Geometry check sheet. Reference: the model listing, model coordinates, mm. A direction names the side the tool comes from. Give positions to 0.01 mm unless a question says otherwise; leave off trailing zeros. Order: outer loops, then holes, each group sorted by start corner. A loop starts at its lowest first (then second) coordinate and runs counter-clockwise, first axis right, second up.
Autodesk Inventor part; units mm, degrees
ref_plane "YZ Plane" through (0, 0, 0) normal (1, 0, 0) x (0, 1, 0)
ref_plane "XZ Plane" through (0, 0, 0) normal (0, 1, 0) x (-1, 0, 0)
ref_plane "XY Plane" through (0, 0, 0) normal (0, 0, 1) x (1, 0, 0)
sketch "スケッチ1" plane through (0, 0, 0) normal (0, 0, 1) x (1, 0, 0)
  circle A0 centre (0, 0) radius 35
  circle A1 centre (0, 0) radius 33
  line L0 (-45, 40) -> (45, 40)
  line L1 (45, 40) -> (45, -40)
  line L2 (45, -40) -> (-45, -40)
  line L3 (-45, -40) -> (-45, 40)
  line L4 (-45, 40) -> (45, -40) construction
  line L5 (45, 40) -> (-45, -40) construction
  dimension "d0" = 70
  dimension "d1" = 66
  dimension "d2" = 90
  dimension "d3" = 80
extrude "押し出し1" add sketch "スケッチ1" along normal blind 3 contours L0 L1 L2 L3
sketch "スケッチ2" plane through (0, 0, 3) normal (0, 0, 1) x (1, 0, 0)
  circle A0 centre (0, 0) radius 35
  circle A1 centre (0, 0) radius 35
  circle A2 centre (0, 0) radius 33
  dimension "d6" = 66
extrude "押し出し2" add sketch "スケッチ2" along normal blind 3 and the other way blind 3
sketch "スケッチ3" plane through (0, 0, 6) normal (0, 0, 1) x (1, 0, 0)
  circle A0 centre (0, 0) radius 33
  circle A1 centre (0, 0) radius 35
extrude "押し出し3" add sketch "スケッチ3" along normal blind 59
sketch "スケッチ4" plane through (0, 0, 65) normal (0, 0, 1) x (1, 0, 0)
  circle A0 centre (0, 0) radius 33
  circle A1 centre (0, 0) radius 35
sketch "スケッチ5" plane through (0, 0, 0) normal (0, 0, -1) x (-1, 0, 0)
  line L0 (-45, 40) -> (-35, 40)
  line L1 (-35, 40) -> (-35, 30)
  line L2 (-35, 30) -> (-45, 30)
  line L3 (-45, 30) -> (-45, 40)
  line L4 (-45, -40) -> (-35, -40)
  line L5 (-35, -40) -> (-35, -30)
  line L6 (-35, -30) -> (-45, -30)
  line L7 (-45, -30) -> (-45, -40)
  line L8 (45, -40) -> (35, -40)
  line L9 (35, -40) -> (35, -30)
  line L10 (35, -30) -> (45, -30)
  line L11 (45, -30) -> (45, -40)
  line L12 (45, 40) -> (35, 40)
  line L13 (35, 40) -> (35, 30)
  line L14 (35, 30) -> (45, 30)
  line L15 (45, 30) -> (45, 40)
  dimension "d13" = 10
  dimension "d14" = 10
  dimension "d15" = 10
  dimension "d16" = 10
  dimension "d17" = 10
  dimension "d18" = 10
  dimension "d19" = 10
hole "穴1" at (35, 30, 0) at (-35, 30, 0) at (-35, -30, 0) at (35, -30, 0) direction (0, 0, 1) diameter 3 depth 8 tip angle 118
sketch "スケッチ6" plane through (0, 0, 0) normal (0, 0, -1) x (-1, 0, 0)
  circle A0 centre (-35, 30) radius 1.5
  circle A1 centre (-35, -30) radius 1.5
  line L0 (-45, -40) -> (45, -40)
  line L1 (-45, 40) -> (0, 40)
  line L2 (0, 40) -> (0, -40)
  line L3 (0, -40) -> (-45, -40)
  line L4 (-45, -40) -> (-45, 40)
extrude "押し出し4" cut sketch "スケッチ6" against normal blind 65
properties part number "知能ロボコン発射口ver2.5"
Item 1: Sectioned sample at D-D (y = -27.5). Enter the section's corners in (x, z), and give its area (3 significant figures).
Reported:
outline: (-45, 0) - (-18.24, 0) - (-18.24, 65) - (-21.65, 65) - (-21.65, 3) - (-45, 3) - close
area: 292 mm2
Item 2: Scan lines: L1, parallel to Y at x = -35, z = 1.45; L2, parallel to Z at x = -26, y = 30.5; L3, parallel to X at y = 30, z = 2.3. Record each from-to range of solid material in increasing order.
Reported:
L1: y = -40 to -31.5, -28.5 to 28.5, 31.5 to 40
L2: z = 0 to 3
L3: x = -45 to -36.5, -33.5 to -13.75
Item 3: Gauge pin test, flat ends, axial feed: pin 1 (5 mm diameter, centred on x = -32.5, z = 10.5, fed in from +Y); pin 2 (3 mm diameter, centred on y = -10.5, z = 42, fed in from -X); pin 3 (12 mm diameter, centred on x = -27.5, z = 32, fed in from +Y); pin 4 (2.5 mm diameter, centred on x = -35, y = 30, fed in from -Z). Record the tip position at first contact, or that the pin passes through.
Reported:
pin 1: stops at y = 18.03
pin 2: stops at x = -33.82
pin 3: stops at y = 27.62
pin 4: passes through
Item 4: Set-up check for faces 1 (the flat face through (-33.1, -2.4, 65)), 2 (the cylindrical face through (-34.99, -0.77, 33.57)): record each of +Z, -Z, +X, -X, +Y, -Y from which the full face is reachable in a straight line by a thin tool's end or side.
Reported:
face 1: +Z, +X, -X, +Y, -Y
face 2: +Z, -X
Item 5: Sectioned sample at A-A (x = -14). Enter the section's corners in (y, z), and give its area (3 significant figures).
Reported:
outline: (-40, 0) - (-29.88, 0) - (-29.88, 65) - (-32.08, 65) - (-32.08, 3) - (-40, 3) - close; (29.88, 0) - (40, 0) - (40, 3) - (32.08, 3) - (32.08, 65) - (29.88, 65) - close
area: 333 mm2
Item 6: Sectioned sample at B-B (y = 30). Enter the section's corners in (x, z), and give its area (3 significant figures).
Reported:
outline: (-45, 0) - (-36.5, 0) - (-36.5, 3) - (-45, 3) - close; (-33.5, 0) - (-13.75, 0) - (-13.75, 65) - (-18.03, 65) - (-18.03, 3) - (-33.5, 3) - close
area: 350 mm2
Item 7: Sectioned sample at C-C (z = 33.5). Enter the section's corners in (x, y).
Reported:
outline: (0, -35) - (0, -33) arc R33 cw to (0, 33) - (0, 35) arc R35 ccw to start
Item 8: Draft check along X on faces 3 (the flat face through (-23, 40, 1)), 4 (the flat face through (-45, -1, 1)), 5 (the cylindrical face through (-32.99, -0.73, 32.04)), 6 (the cylindrical face through (-34.1, 28.8, 1.5)). Enter one of: released by +X, released by -X, zero draft, split by the parting line, or undercut.
Reported:
face 3: zero draft
face 4: released by -X
face 5: released by +X
face 6: undercut
